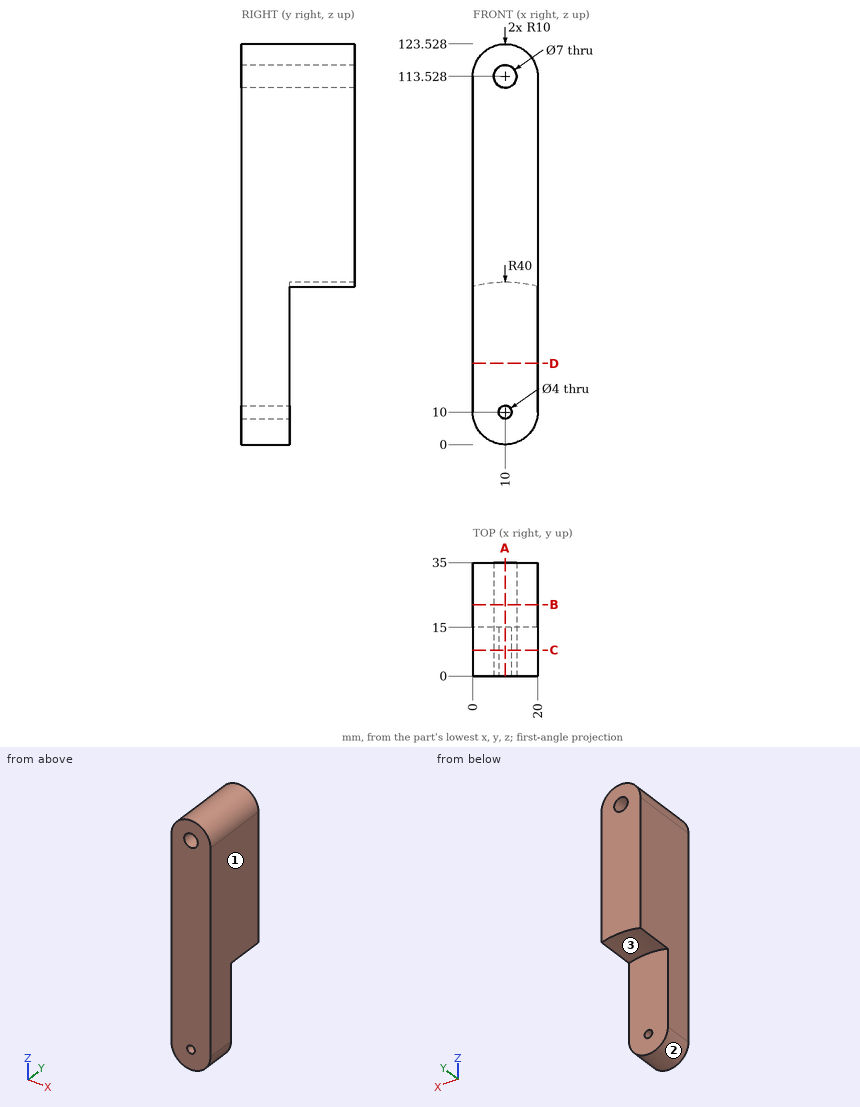
Source: three-view drawing plus pictorial views. Frame: mm from the lowest corner of the part. Give positions to 0.01 mm unless a question says otherwise; leave off trailing zeros. Loops run counter-clockwise (first coordinate to the right, second up) from the corner with the lowest first, then second, coordinate; pieces in that order, holes last. Notation, with made-up numbers: (42.25, -31.75) -> (52.25, -31.75) arc R34 cw to (52.25, 2.25) -> close; hole circle Ø8 at (19, 84.25). An arc over 180 degrees is marked (long way). Use a Markdown table: item, result. Add a question column.
(1) First-contact query: pin 1 Ø6 at (x, z) = (8, 23) entering from +Y; pin 2 Ø5 at (x, y) = (5, 28) entering from -Z; pin 3 Ø1 at (x, y) = (9, 30.5) entering from -Z; pin 4 Ø5.5 at (x, z) = (10, 113.53) entering from -Y. Flat tips, straight axial feed; report the tip coordinate or a pass-through.
(2) Ray query, line 1 (Z direction, x = 10, y = 9.5); line 2 (Z direction, x = 10, y = 16.5); line 3 (Z direction, x = 9.5, y = 3) (1 decimal). Return the intervals inside material, ascending.
(3) Section query D-D (z = 25). Output: boundary loops of the cut face in (x, y), then the cut area to 3 significant figures.
(4) Section query C-C (y = 8). Output: boundary loops of the cut face in (x, z), then the cut area to 3 significant figures.
(5) Section query A-A (x = 10). Output: boundary loops of the cut face in (y, z).
(6) Pull-direction query (X, two-part tool) for the marked faces 1, 2 and 3; classes: +X half, -X half, draft (parallel to the pull), parting line (faces both ways), or undercut.
(7) Section query B-B (y = 22). Output: boundary loops of the cut face in (x, z).
Checked values:
| question | item | result |
|---|---|---|
| 1 | pin 1 | y = 15 |
| 1 | pin 2 | z = 49.29 |
| 1 | pin 3 | z = 49.97 |
| 1 | pin 4 | through |
| 2 | line 1 | 0 to 8, 12 to 110.03, 117.03 to 123.53 |
| 2 | line 2 | 50 to 110.03, 117.03 to 123.53 |
| 2 | line 3 | 0 to 8.1, 11.9 to 110.1, 117 to 123.5 |
| 3 | outline | (0, 0) -> (20, 0) -> (20, 15) -> (0, 15) -> close |
| 3 | area | 300 mm^2 |
| 4 | outline | (0, 10) arc R10 ccw to (20, 10) -> (20, 113.53) arc R10 ccw to (0, 113.53) -> close; hole circle Ø7 at (10, 113.53); hole circle Ø4 at (10, 10) |
| 4 | area | 2,330 mm^2 |
| 5 | outline | (0, 0) -> (15, 0) -> (15, 8) -> (0, 8) -> close; (0, 12) -> (15, 12) -> (15, 50) -> (35, 50) -> (35, 110.03) -> (0, 110.03) -> close; (0, 117.03) -> (35, 117.03) -> (35, 123.53) -> (0, 123.53) -> close |
| 6 | face 1 | +X half |
| 6 | face 2 | parting line |
| 6 | face 3 | undercut |
| 7 | outline | (0, 48.73) arc R40 cw to (20, 48.73) -> (20, 113.53) arc R10 ccw to (0, 113.53) -> close; hole circle Ø7 at (10, 113.53) |
